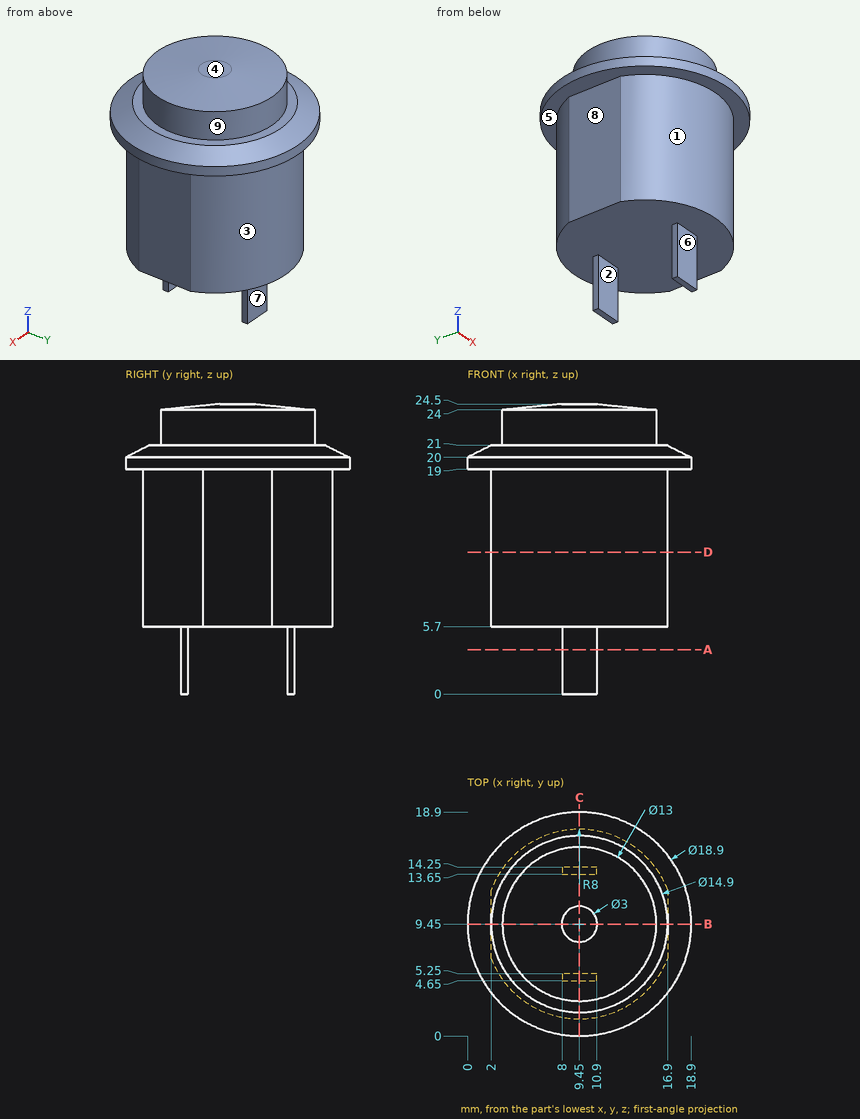
Can you work these out from the drawing? Everything is in mm from the part's minimum corner. A direction names the side the tool comes from. Round coordinates to 2 decimals unless told otherwise and drop trailing zeros. Order: outer loops, then holes, each group sorted by start corner. A loop starts at its lowest first (then second) coordinate and runs counter-clockwise, first axis right, second up. Notation, with made-up numbers: (39, 6) -> (56, 6) arc R14 cw to (56, 16) -> close; hole circle Ø3 at (-15.5, -5). An arc over 180 degrees is marked (long way). Return JSON: item names as keys, results as strings. Group by question number.
1. If we section it at A-A, the plane z = 3.75: Write out the boundary of the cut face in (x, y), then the cut area to 3 significant figures.
2. If we section it at C-C, the plane x = 9.45: Write out the boundary of the cut face in (y, z).
3. We'd pull the mould along Y, two halves only. Please class the marked faces 1, 2, 3 and 4: released by +Y, released by -Y, zero draft, split by the parting line, or undercut.
4. Which directions (+Z, -Z, +X, -X, +Y, -Y) give clear straight access to the entire face, cutting with the end or side of a thin tool? Please do the marked faces 5, 6, 7, 8 and 9.
5. I need wall thicknesses on line 1 (X direction, y = 9.75, z = 7); line 2 (Z direction, x = 5.5, y = 15.5); line 3 (X direction, y = 13, z = 17.5). Which ranges of each line are inside material? Lowest first, please. Write a range as [from, to].
6. Will these pins go through, and if not, where does the flat tip stop? pin 1 (1.5 mm diameter, centred on x = 9.5, z = 2.5, fed in from +Y); pin 2 (4.5 mm diameter, centred on y = 8.5, z = 13.5, fed in from +X); pin 3 (6 mm diameter, centred on x = 4, z = 9.5, fed in from -Y); pin 4 (1.5 mm diameter, centred on x = 6.5, z = 4, fed in from -Y).
7. If we section it at D-D, the plane z = 12: Write out the boundary of the cut face in (x, y).
8. If we section it at B-B, the plane y = 9.45: Write out the boundary of the cut face in (x, z), then the cut area to 3 significant figures.
Output values:
{
 "1": {"outline": "(8, 4.65) -> (10.9, 4.65) -> (10.9, 5.25) -> (8, 5.25) -> close; (8, 13.65) -> (10.9, 13.65) -> (10.9, 14.25) -> (8, 14.25) -> close", "area": "3.48 mm²"},
 "2": {"outline": "(0, 19) -> (1.45, 19) -> (1.45, 5.7) -> (4.65, 5.7) -> (4.65, 0) -> (5.25, 0) -> (5.25, 5.7) -> (13.65, 5.7) -> (13.65, 0) -> (14.25, 0) -> (14.25, 5.7) -> (17.45, 5.7) -> (17.45, 19) -> (18.9, 19) -> (18.9, 20) -> (16.9, 21) -> (15.95, 21) -> (15.95, 24) -> (10.95, 24.5) -> (7.95, 24.5) -> (2.95, 24) -> (2.95, 21) -> (2, 21) -> (0, 20) -> close"},
 "3": {"face 1": "released by -Y", "face 2": "undercut", "face 3": "released by +Y", "face 4": "zero draft"},
 "4": {"face 5": "-Z", "face 6": "-Z, +X, -X, -Y", "face 7": "-Z, +X, -X, +Y", "face 8": "-Z, -X, +Y, -Y", "face 9": "+Z"},
 "5": {"line 1": "[2, 16.9]", "line 2": "[5.7, 21]", "line 3": "[2.28, 16.62]"},
 "6": {"pin 1": "y = 14.25", "pin 2": "x = 16.9", "pin 3": "y = 1.83", "pin 4": "through"},
 "7": {"outline": "(2, 6.53) arc R8 ccw to (16.9, 6.53) -> (16.9, 12.37) arc R8 ccw to (2, 12.37) -> close"},
 "8": {"outline": "(0, 19) -> (2, 19) -> (2, 5.7) -> (16.9, 5.7) -> (16.9, 19) -> (18.9, 19) -> (18.9, 20) -> (16.9, 21) -> (15.95, 21) -> (15.95, 24) -> (10.95, 24.5) -> (7.95, 24.5) -> (2.95, 24) -> (2.95, 21) -> (2, 21) -> (0, 20) -> close", "area": "277 mm²"}
}
